Input: part model. Units: mm. Frame: model coordinates. A direction names the side the tool comes from. Round coordinates to 2 decimals unless told otherwise and drop trailing zeros. Write each loop counter-clockwise with the first axis right and the second up, starting at its lowest first coordinate (ties: lowest second). Pieces come first, ordered by that corner, then holes. Notation, with made-up numbers: M -12.75,60.25 L 44.25,60.25 A16 ccw 44.25,69.25 Z; hole C 85.25,45 d8. An arc over 180 degrees is marked long. Write each question's results on one line, items separated by ' | '. Start each with the question number.
```python
from build123d import *

# Parameters (mm, degrees)
SKETCH_1_R            = 3.1
SKETCH_1_R_2          = 7.6
SKETCH_1_R_3          = 6.1
EXTRUDE_1_DEPTH       = 4
CUT_EXTRUDE_1_DEPTH   = 4
FILLET_1_R            = 2
FILLET_2_R            = 5
CUT_EXTRUDE_START     = -10
CUT_EXTRUDE_2_DEPTH   = 10
CHAMFER_START         = -75.71880289
CHAMFER_2_OUTLINE_W   = 9.932436379
CHAMFER_2_OUTLINE_H   = 4
CHAMFER_2_DEPTH       = 0.082131492
CHAMFER_START_2       = -75.636671398
CHAMFER_2_2_OUTLINE_W = 9.932436379
CHAMFER_2_2_OUTLINE_H = 4
CHAMFER_2_2_DEPTH     = 1.179418361
FILLET_4_R            = 15
FILLET_5_R            = 10


with BuildPart() as part:
    # 草图1 → 凸台-拉伸1 (new body)
    with BuildSketch(Plane.XY):
        with BuildLine():
            Line((-47.242305659, 68.18165139), (-17.969613961, -2.672844027))
            ThreePointArc((-17.969613961, -2.672844027), (-15.391663642, -5.818501018), (-11.5, -7))
            Line((-11.5, -7), (11.5, -7))
            ThreePointArc((11.5, -7), (16.568173397, -4.828417796), (18.491788179, 0.338966167))
            Line((18.491788179, 0.338966167), (14.98240324, 72.726356073))
            ThreePointArc((14.98240324, 72.726356073), (9.608039696, 83.518922397), (-1.973684211, 86.869585423))
            Line((-1.973684211, 86.869585423), (-39.315789474, 81.913056948))
            ThreePointArc((-39.315789474, 81.913056948), (-46.660613019, 76.999378175), (-47.242305659, 68.18165139))
        make_face()
        with Locations((11.5, 0)):
            Circle(SKETCH_1_R, mode=Mode.SUBTRACT)
        with Locations((-11.5, 0)):
            Circle(SKETCH_1_R, mode=Mode.SUBTRACT)
        with Locations((0, 72)):
            Circle(SKETCH_1_R_2, mode=Mode.SUBTRACT)
        with Locations((-38, 72)):
            Circle(SKETCH_1_R_3, mode=Mode.SUBTRACT)
    extrude(amount=EXTRUDE_1_DEPTH)

    # 草图2 → 切除-拉伸1 (cut)
    with BuildSketch(Plane.XY.offset(4)):
        Polygon((0, 60.4), (-14, 8), (14, 8), align=None)
        Polygon((-35.991267369, 61.9), (-7.879846422, 61.9), (-18.919878801, 20.578735952), align=None)
    extrude(amount=-CUT_EXTRUDE_1_DEPTH, mode=Mode.SUBTRACT)

    # 圆角1
    fillet_1_edges = [part.edges().sort_by_distance(p)[0] for p in [
        (-18.919878801, 20.578735952, 2),
        (-35.991267369, 61.9, 2),
        (-7.879846422, 61.9, 2),
        (0, 60.4, 2),
        (-14, 8, 2),
    ]]
    fillet(fillet_1_edges, radius=FILLET_1_R)

    # 圆角2
    fillet_2_edges = [part.edges().sort_by_distance(p)[0] for p in [
        (14, 8, 2),
    ]]
    fillet(fillet_2_edges, radius=FILLET_2_R)

    # 草图3 → 切除-拉伸2 (cut)
    with BuildSketch(Plane.XY.offset(4).offset(CUT_EXTRUDE_START)):
        with BuildLine():
            Line((-30.07293559, 78.096035584), (-12.403974557, 80.441289229))
            ThreePointArc((-12.403974557, 80.441289229), (-8.018810771, 84.681191682), (-2.308312161, 86.825169261))
            Line((-2.308312161, 86.825169261), (-39.315789474, 81.913056948))
            ThreePointArc((-39.315789474, 81.913056948), (-34.182978636, 81.242853883), (-30.07293559, 78.096035584))
        make_face()
    extrude(amount=CUT_EXTRUDE_2_DEPTH, mode=Mode.SUBTRACT)

    # 倒角1
    # the kernel refuses this chamfer: 10 mm, written as the material it adds along each edge
    with BuildSketch(Plane(origin=(-30.07293559, 78.096035584, 0), x_dir=(0.9913056948335455, 0.13157894736842105, 0), z_dir=(0, 0, 1))) as chamfer_1_piece_1:
        with BuildLine():
            Line((7.475531418, -0.121000067), (-3.274957131, 3.290873048))
            Line((-3.274957131, 3.290873048), (-3.390288264, 3.127475588))
            ThreePointArc((-3.390288264, 3.127475588), (-1.542012582, 1.735773049), (-0.173205081, -0.1))
            Line((-0.173205081, -0.1), (0, -0.2))
            ThreePointArc((0, -0.2), (3.737765709, -0.2), (7.475531418, -0.321000067))
            Line((7.475531418, -0.321000067), (7.475531418, -0.121000067))
        make_face()
    extrude(amount=4)

    # 倒角2: read off the stored shape, not the designer's step
    # 倒角2 outline → 倒角2 (cut)
    with BuildSketch(Plane(origin=(0, 0, 0), x_dir=(0.8432639594677482, 0.5374996694536432, 0), z_dir=(0.5374996694536432, -0.8432639594677483, 0)).offset(CHAMFER_START)):
        with Locations((35.301502575, 2)):
            Rectangle(CHAMFER_2_OUTLINE_W, CHAMFER_2_OUTLINE_H)
    extrude(amount=CHAMFER_2_DEPTH, mode=Mode.SUBTRACT)

    # Chamfer 2 2 outline → Chamfer 2 2 (add)
    with BuildSketch(Plane(origin=(0, 0, 0), x_dir=(0.8432639594677482, 0.5374996694536432, 0), z_dir=(0.5374996694536432, -0.8432639594677483, 0)).offset(CHAMFER_START_2)):
        with Locations((35.301502575, 2)):
            Rectangle(CHAMFER_2_2_OUTLINE_W, CHAMFER_2_2_OUTLINE_H)
    extrude(amount=CHAMFER_2_2_DEPTH)

    # 圆角4
    fillet_4_edges = [part.edges().sort_by_distance(p)[0] for p in [
        (-23.040343668, 79.029492385, 2),
        (-33.358562851, 80.857599065, 2),
        (-15.074033853, 80.086884334, 2),
    ]]
    fillet(fillet_4_edges, radius=FILLET_4_R)

    # 圆角5
    fillet_5_edges = [part.edges().sort_by_distance(p)[0] for p in [
        (-6.698368225, 85.425565604, 2),
    ]]
    fillet(fillet_5_edges, radius=FILLET_5_R)


solid = part.part
```
1. Cut plane C-C on x = -16. Output: boundary loops of the cut face in (y, z), and give its area (3 significant figures).
2. Cut plane D-D on y = 74. Output: boundary loops of the cut face in (x, z).
3. Access query for faces 5 (the face through (-4.029, 86.453, 1.972)), 6 (the face through (-15.241, 80.412, 2.028)), 7 (the face through (7.198, 33.457, 2.028)). Directions: +Z, -Z, +X, -X, +Y, -Y. A direction counts if a zero-diameter tool reaches every point of the face in a straight line with its end or side. Return the directions, or none.
4. Cut plane A-A on x = 1. Output: boundary loops of the cut face in (y, z), and give its area (3 significant figures).
5. Contact query for flat-ended pins moving along their axis: P1, Ø2, axis at x = 2, z = 3, coming from the +Y side; P2, Ø7, axis at x = -11.5, y = 0, coming from the -Z side; P3, Ø2, axis at x = 7, z = 3, coming from the +Y side; P4, Ø2, axis at x = -17, z = 2, coming from the -Y side. Output: stop coordinate, or through.
6. Draft query along X for faces 1 (the face through (-19.57, 79.49, 1.97)), 2 (the face through (-22, 61.9, 2)), 3 (the face through (-32.81, 33.25, 1.97)), 4 (the face through (16.5, -4.9, 2)). Return one class per face: +X half, -X half, draft (parallel to the pull), parting line (faces both ways), or undercut.
7. Line query: L1, parallel to Y at x = 0, z = 1.85; L2, parallel to X at y = -1.5, z = 1.85; L3, parallel to X at y = 33.5, z = 1.05. Output: solid intervals per line, ascending. Write a range as from..to.
8. Cut plane B-B on z = 2.55. Give the number of separate pieces and of enclosed holes in the cut face, and give its area (3 significant figures).
Answers follow:
1) outline: M -5.36,0 L 31.51,0 L 31.51,4 L -5.36,4 Z; M 61.9,0 L 80.16,0 L 80.16,4 L 61.9,4 Z | area: 221 mm2
2) outline: M -47.8,0 L -43.76,0 L -43.76,4 L -47.8,4 Z; M -32.24,0 L -7.33,0 L -7.33,4 L -32.24,4 Z; M 7.33,0 L 14.87,0 L 14.87,4 L 7.33,4 Z
3) face 5: +Z, -Z, -X, +Y | face 6: +Z, -Z, +Y | face 7: +Z, -Z
4) outline: M -7,0 L 8,0 L 8,4 L -7,4 Z; M 54.38,0 L 64.47,0 L 64.47,4 L 54.38,4 Z; M 79.53,0 L 86.97,0 L 86.97,4 L 79.53,4 Z | area: 130 mm2
5) P1: stops at y = 86.97 | P2: stops at z = 0 | P3: stops at y = 85.75 | P4: stops at y = -5.36
6) face 1: undercut | face 2: undercut | face 3: -X half | face 4: +X half
7) L1: y = -7..8, 54.65..64.4, 79.6..87 | L2: x = -18.45..-14.21, -8.79..8.79, 14.21..18.34 | L3: x = -32.91..-24.26, -15.47..-7.19, 7.19..16.88
8) separate pieces: 1 | enclosed holes: 6 | area: 2,880 mm2
